Could you check a few things on this model? Use its own coordinates, in mm. A direction names the side the tool comes from. Give positions to 0.01 mm unless a question says otherwise; leave off trailing zeros. Loops run counter-clockwise (first coordinate to the right, second up) from the corner with the lowest first, then second, coordinate; pieces in that order, holes last. Notation, with made-up numbers: (29.25, 62) - (76.25, 62) arc R12 cw to (76.25, 75) - close; hole circle Ø3 at (31.5, 31). An arc over 180 degrees is marked (long way). One line per item, written item: value. Start each with the question number.
Q1. I'm going to push flat-ended pins straight in: P1, Ø3, axis at y = 102.5, z = 227, coming from the -X side; P2, Ø4, axis at y = 288.5, z = 1142.5, coming from the +X side. Where does each tip first touch, or does it pass through?
Q2. For faces 4 (the face through (200, 0, 814)), 5 (the face through (216, 806.45, 814)), which set-ups out of +Z, -Z, +X, -X, +Y, -Y let a thin tool reach every point of the face, with its end or its side?
Q3. I want a section at C-C (z = 233.5). Please give me the cut outline in (x, y).
Q4. If I drill on line 1 (Y direction, x = 336, z = 1454); line 2 (Z direction, x = 204, y = 546); line 3 (Y direction, x = 389, z = 916.5), over which ranges is the centre line in solid material (lowest first)? Write a range as from..to.
Q5. I want a section at D-D (y = 716.5). Please give me the cut outline in (x, z).
Q6. If we mould it in two halves opening along Z, with no side actions, what happens to faces 1 (the face through (0, 401, 814)), 2 (the face through (216, 412, 6.35)), 3 (the face through (200, 412, 1651))? For each: released by +Z, released by -Z, zero draft, split by the parting line, or undercut.
Q7. I want a section at B-B (y = 203). Please give me the cut outline in (x, z), then the cut area to 3 significant figures.
Q8. I want a section at A-A (x = 259.5). Please give me the cut outline in (y, z), then the cut area to 3 significant figures.
```python
from build123d import *

# Parameters (mm, degrees)
F0_W     = 406.4
F0_H     = 812.8
F1_DEPTH = 1651
F2_T     = -6.35
F3_DEPTH = 25.4
F4_W     = 190.5
F4_H     = 190.5
F5_DEPTH = 304.8


with BuildPart() as f1:
    # F0 (on Top) → F1 (new body)
    with BuildSketch(Plane.XY):
        with Locations((203.2, 406.4)):
            Rectangle(F0_W, F0_H)
    extrude(amount=F1_DEPTH)

    # F2
    f2_openings = [f1.faces().sort_by_distance(p)[0] for p in [
        (406.4, 406.4, 825.5),
    ]]
    offset(amount=F2_T, openings=f2_openings)

    # F3 (add): a face of the model
    f3_faces = [f1.faces().sort_by_distance(p)[0] for p in [
        (6.35, 406.4, 825.5),
    ]]
    extrude(f3_faces, amount=F3_DEPTH)

    # F4 (on face) → F5 (join)
    with BuildSketch(Plane.YZ.offset(31.75)):
        with Locations((228.6, 1422.4)):
            Rectangle(F4_W, F4_H)
    extrude(amount=F5_DEPTH)


solid = f1.part
```
Worked answers:
1. P1: stops at x = 0
1. P2: stops at x = 31.75
2. face 4: +Z, -Z, +X, -X, -Y
2. face 5: +X
3. outline: (0, 0) - (406.4, 0) - (406.4, 6.35) - (31.75, 6.35) - (31.75, 806.45) - (406.4, 806.45) - (406.4, 812.8) - (0, 812.8) - close
4. line 1: y = 0..6.35, 133.35..323.85, 806.45..812.8
4. line 2: z = 0..6.35, 1644.65..1651
4. line 3: y = 0..6.35, 806.45..812.8
5. outline: (0, 0) - (406.4, 0) - (406.4, 6.35) - (31.75, 6.35) - (31.75, 1644.65) - (406.4, 1644.65) - (406.4, 1651) - (0, 1651) - close
6. face 1: zero draft
6. face 2: undercut
6. face 3: released by +Z
7. outline: (0, 0) - (406.4, 0) - (406.4, 6.35) - (31.75, 6.35) - (31.75, 1327.15) - (336.55, 1327.15) - (336.55, 1517.65) - (31.75, 1517.65) - (31.75, 1644.65) - (406.4, 1644.65) - (406.4, 1651) - (0, 1651) - close
7. area: 115,000 mm²
8. outline: (0, 0) - (812.8, 0) - (812.8, 1651) - (0, 1651) - close; (133.35, 1327.15) - (323.85, 1327.15) - (323.85, 1517.65) - (133.35, 1517.65) - close; hole (6.35, 6.35) - (806.45, 6.35) - (806.45, 1644.65) - (6.35, 1644.65) - close
8. area: 67,400 mm²
